```python
from build123d import *

# Parameters (mm, degrees)
SKETCH1_W           = 40
SKETCH1_H           = 20
BOSS_EXTRUDE1_DEPTH = 40
CUT_EXTRUDE1_DEPTH  = 40
CUT_EXTRUDE2_DEPTH  = 40
CUT_EXTRUDE3_DEPTH  = 10
CUT_EXTRUDE4_DEPTH  = 10
BOSS_EXTRUDE2_DEPTH = 10


with BuildPart() as part:
    # Sketch1 → Boss-Extrude1 (new body)
    with BuildSketch(Plane.XY):
        with BuildLine():
            Line((0, 20), (40, 20))
            ThreePointArc((40, 20), (20, 40), (0, 20))
        make_face()
        with Locations((20, 10)):
            Rectangle(SKETCH1_W, SKETCH1_H)
    extrude(amount=BOSS_EXTRUDE1_DEPTH)

    # Sketch2 → Cut-Extrude1 (cut)
    with BuildSketch(Plane(origin=(0, 0, 0), x_dir=(1, 0, 0), z_dir=(0, 1, 0))):
        with BuildLine():
            Line((0, -20), (0, -40))
            Line((0, -40), (20, -40))
            ThreePointArc((20, -40), (5.857864, -34.142136), (0, -20))
        make_face()
        with BuildLine():
            ThreePointArc((40, -20), (34.142136, -34.142136), (20, -40))
            Line((20, -40), (40, -40))
            Line((40, -40), (40, -20))
        make_face()
    extrude(amount=CUT_EXTRUDE1_DEPTH, mode=Mode.SUBTRACT)

    # Sketch3 → Cut-Extrude2 (cut)
    with BuildSketch(Plane(origin=(0, 0, 0), x_dir=(0, 0, -1), z_dir=(1, 0, 0))):
        Polygon((-40, 20), (-20, 40), (-40, 40), align=None)
    extrude(amount=CUT_EXTRUDE2_DEPTH, mode=Mode.SUBTRACT)

    # Sketch4 → Cut-Extrude3 (cut)
    with BuildSketch(Plane(origin=(0, 0, 0), x_dir=(-1, 0, 0), z_dir=(0, 0, -1))):
        with BuildLine():
            Line((-40, 20), (-20, 40))
            ThreePointArc((-20, 40), (-34.142136, 34.142136), (-40, 20))
        make_face()
        with BuildLine():
            ThreePointArc((0, 20), (-5.857864, 34.142136), (-20, 40))
            Line((-20, 40), (0, 20))
        make_face()
    extrude(amount=-CUT_EXTRUDE3_DEPTH, mode=Mode.SUBTRACT)

    # Sketch5 → Cut-Extrude4 (cut)
    with BuildSketch(Plane.XY.offset(10)):
        Polygon((40, 20), (40, 40), (0, 20), align=None)
        with BuildLine():
            ThreePointArc((32, 36), (11.055728, 37.888544), (0, 20))
            Line((0, 20), (32, 36))
        make_face()
    extrude(amount=CUT_EXTRUDE4_DEPTH, mode=Mode.SUBTRACT)

    # Sketch7 → Boss-Extrude2 (add)
    with BuildSketch(Plane(origin=(0, 0, 20), x_dir=(-1, 0, 0), z_dir=(0, 0, -1))):
        with BuildLine():
            Line((0, 20), (-34.142136, 34.142136))
            ThreePointArc((-34.142136, 34.142136), (-38.477591, 27.653669), (-40, 20))
            Line((-40, 20), (0, 20))
        make_face()
    extrude(amount=BOSS_EXTRUDE2_DEPTH)


solid = part.part
```
Source: CAD feature listing. Evaluate the final solid. Frame: model axes, mm. A direction names the side the tool comes from. Round coordinates to 2 decimals unless told otherwise and drop trailing zeros. Write each loop counter-clockwise with the first axis right and the second up, starting at its lowest first coordinate (ties: lowest second). Pieces come first, ordered by that corner, then holes. Notation, with made-up numbers: M -6,-23 L 35,-23 A31 cw 35,10 Z; hole C -30,53 d1. An arc over 180 degrees is marked long. Use CSV: the item, a comma, the result in double quotes. Start each with the question number.
Q1. Access query for faces 1 (the face through (20, 30, 30)), 2 (the face through (36, 29, 10)), 3 (the face through (10, 30, 5)), 4 (the face through (16.83, 26.97, 15.07)). Directions: +Z, -Z, +X, -X, +Y, -Y. A direction counts if a zero-diameter tool reaches every point of the face in a straight line with its end or side. Return the directions, or none.
Q2. Cut plane A-A on x = 17. Output: boundary loops of the cut face in (y, z).
Q3. Pull-direction query (Z, two-part tool) for faces 5 (the face through (13, 32, 20)), 6 (the face through (20, 0, 20)), 7 (the face through (20, 16, 0)); classes: +Z half, -Z half, draft (parallel to the pull), parting line (faces both ways), or undercut.
Q4. Cut plane D-D on x = 30. Output: boundary loops of the cut face in (y, z), plus the area to 3 significant figures.
Q5. Cut plane B-B on z = 4. Output: boundary loops of the cut face in (x, y).
Q6. Line query: line 1 (X direction, y = 11.5, z = 21); line 2 (Z direction, x = 31, y = 22.5); line 3 (Z direction, x = 21.5, y = 33.5). Output: solid intervals per line, ascending. Write a range as from..to.
Q7. First-contact query: P1, Ø12, axis at x = 7, y = 35, coming from the -Z side; P2, Ø3, axis at x = 8.5, z = 23.5, coming from the +Y side; P3, Ø12, axis at x = 33.5, z = 33.5, coming from the +Y side; P4, Ø4, axis at y = 24, z = 14.5, coming from the -X side. Flat tips, straight axial feed; report the tip coordinate or a pass-through.
Q8. Cut plane C-C on y = 6. Output: boundary loops of the cut face in (x, z).
Results found:
1,face 1,"+Z, +X, -X, +Y"
1,face 2,"-Z, +X, +Y"
1,face 3,"-Z, -X, +Y"
1,face 4,"-X, +Y"
2,outline,"M 0,0 L 37,0 L 37,10 L 27.04,10 L 27.04,20 L 39.77,20 L 39.77,20.23 L 20.23,39.77 L 0,39.77 Z"
3,face 5,"undercut"
3,face 6,"draft"
3,face 7,"-Z half"
4,outline,"M 0,0 L 30,0 L 30,10 L 32.43,10 L 32.43,20 L 37.32,20 L 37.32,22.68 L 22.68,37.32 L 0,37.32 Z"
4,area,"1,160 mm^2"
5,outline,"M 0,0 L 40,0 L 40,20 L 20,40 L 0,20 Z"
6,line 1,"0.03..39.97"
6,line 2,"0..36.7"
6,line 3,"0..10, 20..26.5"
7,P1,"z = 0"
7,P2,"y = 37.21"
7,P3,"y = 32.5"
7,P4,"x = 4.83"
8,outline,"M 0,0 L 40,0 L 40,20 A20 ccw 20,40 A20 ccw 0,20 Z"
